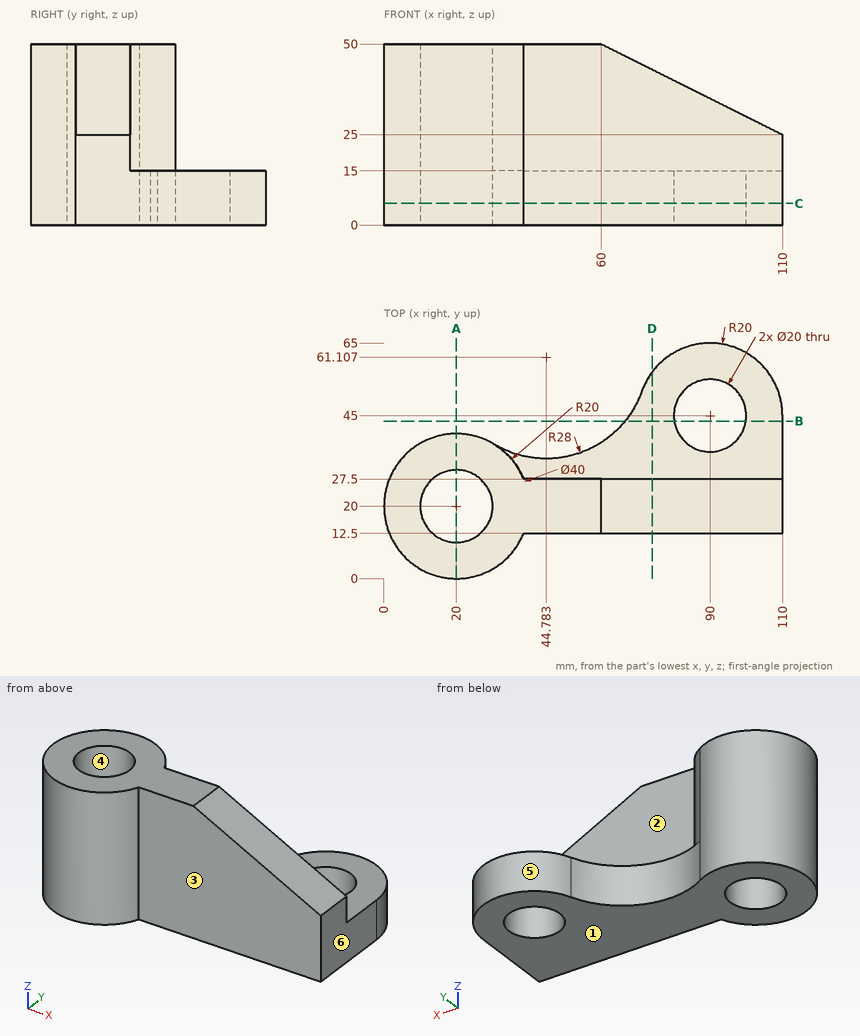
Part print with two shaded views. Sizes in mm from the minimum x, y, z corner. A direction names the side the tool comes from. Give positions to 0.01 mm unless a question says otherwise; leave off trailing zeros. Loops run counter-clockwise (first coordinate to the right, second up) from the corner with the lowest first, then second, coordinate; pieces in that order, holes last. Notation, with made-up numbers: (-38, 63) -> (-2, 63) arc R24 ccw to (-2, 75) -> close; hole circle Ø5 at (-23, 30). An arc over 180 degrees is marked (long way). One line per question, with ' | ' between items.
Q1. Drill centre lines: line 1 along Y through (x, z) = (20, 27); line 2 along Y through (x, z) = (90, 11.25); line 3 along Y through (x, z) = (83, 29). Where is each one in solid material? Low to high. Write a range as [from, to].
Filled sheet:
line 1: y = [0, 10], [30, 40] | line 2: y = [12.5, 35], [55, 65] | line 3: y = [12.5, 27.5]
Q2. Cut at D-D, the plane x = 74. Write the cut outline in (y, z), plus the area to 3 significant figures.
Filled sheet:
outline: (12.5, 0) -> (57, 0) -> (57, 15) -> (27.5, 15) -> (27.5, 43) -> (12.5, 43) -> close | area: 1,090 mm²
Q3. Cut at A-A, the plane x = 20. Write the cut outline in (y, z).
Filled sheet:
outline: (0, 0) -> (10, 0) -> (10, 50) -> (0, 50) -> close; (30, 0) -> (40, 0) -> (40, 50) -> (30, 50) -> close
Q4. Pull direction Y, two halves, no side cores. Call the marked faces 3, 4, 5 and 6: pulls with the +Y half, pulls with the -Y half, needs draft (parallel to the pull), parting line crosses it, or undercut.
Filled sheet:
face 3: pulls with the -Y half | face 4: undercut | face 5: pulls with the +Y half | face 6: needs draft
Q5. Drop flat-ended pins along their axis: pin 1 (3 mm diameter, centred on y = 17, z = 38.5, fed in from -X); pin 2 (2 mm diameter, centred on y = 54, z = 9.5, fed in from +X); pin 3 (3 mm diameter, centred on x = 35, z = 6.5, fed in from -Y). Give the stop position or say it passes through.
Filled sheet:
pin 1: stops at x = 0.06 | pin 2: stops at x = 108.33 | pin 3: stops at y = 5.24
Q6. Cut at C-C, the plane z = 6. Write the cut outline in (x, y), plus the area to 3 significant figures.
Filled sheet:
outline: (30.33, 37.13) arc R20 ccw (long way) to (38.54, 12.5) -> (110, 12.5) -> (110, 45) arc R20 ccw to (71.16, 51.71) arc R28 cw to start; hole circle Ø20 at (20, 20); hole circle Ø20 at (90, 45) | area: 3,320 mm²
Q7. Cut at B-B, the plane y = 43.5. Write the cut outline in (x, z), plus the area to 3 significant figures.
Filled sheet:
outline: (66.55, 0) -> (80.11, 0) -> (80.11, 15) -> (66.55, 15) -> close; (99.89, 0) -> (110, 0) -> (110, 15) -> (99.89, 15) -> close | area: 355 mm²
Q8. Tool access for the marked faces 1 and 2: list every direction of +Z, -Z, +X, -X, +Y, -Y with a clear straight run to the whole face (end or side of a thin tool).
Filled sheet:
face 1: -Z, +X, -X, +Y, -Y | face 2: +Z, +X, +Y
